from build123d import *

# Parameters (mm, degrees)
F1_DEPTH     = 1.524
F2_T1_DEPTH  = 78.232
F2_T3_DEPTH  = 46.482
F2_T6_ANGLE  = 90
F2_T8_ANGLE  = 90
F2_T10_ANGLE = 90
F2_T12_ANGLE = 90


# Not quite as in the source:
# - a fillet or chamfer that OpenCascade refuses, or shapes differently, is made with other operations: its cross-section is extruded or revolved along the edge and cut away or added


with BuildPart() as f1:
    # F0 (on Front) → F1 (new body)
    with BuildSketch(Plane.XZ):
        with BuildLine():
            Line((-23.241, -47.498), (23.241, -47.498))
            ThreePointArc((23.241, -47.498), (29.1679690399, -45.0429690399), (31.623, -39.116))
            Line((31.623, -39.116), (31.623, 39.116))
            ThreePointArc((31.623, 39.116), (29.1679690399, 45.0429690399), (23.241, 47.498))
            Line((23.241, 47.498), (-23.241, 47.498))
            ThreePointArc((-23.241, 47.498), (-29.1679690399, 45.0429690399), (-31.623, 39.116))
            Line((-31.623, 39.116), (-31.623, -39.116))
            ThreePointArc((-31.623, -39.116), (-29.1679690399, -45.0429690399), (-23.241, -47.498))
        make_face()
    extrude(amount=F1_DEPTH)

    # F2: fillet of radius 7.62 on 1 edges, made by hand

    # F2_s2 → F2_t1 (cut)
    with BuildSketch(Plane.XY.offset(-39.116)):
        with BuildLine():
            ThreePointArc((-31.623, 0), (-29.460655577, -1.1329667311), (-27.051, -1.524))
            Line((-27.051, -1.524), (-31.623, -1.524))
            Line((-31.623, -1.524), (-31.623, 0))
        make_face()
        with BuildLine():
            ThreePointArc((31.623, 0), (29.460655577, -1.1329667311), (27.051, -1.524))
            Line((27.051, -1.524), (31.623, -1.524))
            Line((31.623, -1.524), (31.623, 0))
        make_face()
    extrude(amount=F2_T1_DEPTH, mode=Mode.SUBTRACT)

    # F2_s4 → F2_t3 (cut)
    with BuildSketch(Plane.YZ.offset(-23.241)):
        with BuildLine():
            ThreePointArc((0, -47.498), (-1.1329667311, -45.335655577), (-1.524, -42.926))
            Line((-1.524, -42.926), (-1.524, -47.498))
            Line((-1.524, -47.498), (0, -47.498))
        make_face()
        with BuildLine():
            ThreePointArc((0, 47.498), (-1.1329667311, 45.335655577), (-1.524, 42.926))
            Line((-1.524, 42.926), (-1.524, 47.498))
            Line((-1.524, 47.498), (0, 47.498))
        make_face()
    extrude(amount=F2_T3_DEPTH, mode=Mode.SUBTRACT)

    # F2_s5 → F2_t6 (revolve, cut)
    with BuildSketch(Plane.YZ.offset(-23.241)):
        with BuildLine():
            ThreePointArc((0, 47.498), (-1.1329667311, 45.335655577), (-1.524, 42.926))
            Line((-1.524, 42.926), (-1.524, 47.498))
            Line((-1.524, 47.498), (0, 47.498))
        make_face()
    revolve(axis=Axis((-23.241, -1.524, 39.116), (0, -1, 0)), revolution_arc=F2_T6_ANGLE, mode=Mode.SUBTRACT)

    # F2_s7 → F2_t8 (revolve, cut)
    with BuildSketch(Plane.XY.offset(-39.116)):
        with BuildLine():
            ThreePointArc((-31.623, 0), (-29.460655577, -1.1329667311), (-27.051, -1.524))
            Line((-27.051, -1.524), (-31.623, -1.524))
            Line((-31.623, -1.524), (-31.623, 0))
        make_face()
    revolve(axis=Axis((-23.241, -1.524, -39.116), (0, -1, 0)), revolution_arc=F2_T8_ANGLE, mode=Mode.SUBTRACT)

    # F2_s9 → F2_t10 (revolve, cut)
    with BuildSketch(Plane.YZ.offset(23.241)):
        with BuildLine():
            ThreePointArc((0, -47.498), (-1.1329667311, -45.335655577), (-1.524, -42.926))
            Line((-1.524, -42.926), (-1.524, -47.498))
            Line((-1.524, -47.498), (0, -47.498))
        make_face()
    revolve(axis=Axis((23.241, -1.524, -39.116), (0, -1, 0)), revolution_arc=F2_T10_ANGLE, mode=Mode.SUBTRACT)

    # F2_s11 → F2_t12 (revolve, cut)
    with BuildSketch(Plane.XY.offset(39.116)):
        with BuildLine():
            ThreePointArc((31.623, 0), (29.460655577, -1.1329667311), (27.051, -1.524))
            Line((27.051, -1.524), (31.623, -1.524))
            Line((31.623, -1.524), (31.623, 0))
        make_face()
    revolve(axis=Axis((23.241, -1.524, 39.116), (0, -1, 0)), revolution_arc=F2_T12_ANGLE, mode=Mode.SUBTRACT)


solid = f1.part
Could you check a few things on this model? Use its own coordinates, in mm. Give positions to 0.01 mm unless a question says otherwise; leave off trailing zeros. Order: outer loops, then holes, each group sorted by start corner. A loop starts at its lowest first (then second) coordinate and runs counter-clockwise, first axis right, second up. Notation, with made-up numbers: (-17, 40.25) - (32, 40.25) arc R21 ccw to (32, 46.25) - close; hole circle Ø3 at (-25, 77). An arc over 180 degrees is marked (long way). Return JSON: item names as keys, results as strings. Group by question number.
Q1. Suppose I cut it at A-A, the plane x = 4. Please give me the cut outline in (y, z).
Q2. Please list where these lines run through material, in increasing order: line 1 along Y through (x, z) = (1.5, 43.5); line 2 along X through (y, z) = (-0.2, 3.5); line 3 along Z through (x, y) = (0.5, -0.7). Write a range as [from, to].
Q3. Suppose I cut it at B-B, the plane z = -26. Please give me the cut outline in (x, y), and give its area (3 significant figures).
Resolved:
{
 "1": {"outline": "(-1.52, -42.93) arc R7.62 ccw to (0, -47.5) - (0, 47.5) arc R7.62 ccw to (-1.52, 42.93) - close"},
 "2": {"line 1": "y = [-1.5, 0]", "line 2": "x = [-31.34, 31.34]", "line 3": "z = [-46.37, 46.37]"},
 "3": {"outline": "(-31.62, 0) arc R7.62 ccw to (-27.05, -1.52) - (27.05, -1.52) arc R7.62 ccw to (31.62, 0) - close", "area": "91.9 mm2"}
}
